from build123d import *

# Parameters (mm, degrees)
CROQUIS1_R              = 25.4
CROQUIS1_R_2            = 23.4
SALIENTE_EXTRUIR1_DEPTH = 1350
CROQUIS2_R              = 4
CROQUIS2_W              = 2520
CROQUIS2_H              = 10
CORTAR_EXTRUIR1_DEPTH   = 1351.477811739


with BuildPart() as part:
    # Croquis1 → Saliente-Extruir1 (new, symmetric)
    with BuildSketch(Plane(origin=(0, 0, 0), x_dir=(0, 0, -1), z_dir=(1, 0, 0))):
        Circle(CROQUIS1_R)
        Circle(CROQUIS1_R_2, mode=Mode.SUBTRACT)
    extrude(amount=SALIENTE_EXTRUIR1_DEPTH, both=True)

    # Croquis2 → Cortar-Extruir1 (cut, through all)
    with BuildSketch(Plane.XY):
        with Locations((-1339.465777124, 0)):
            Circle(CROQUIS2_R)
        Rectangle(CROQUIS2_W, CROQUIS2_H)
    extrude(amount=-CORTAR_EXTRUIR1_DEPTH, mode=Mode.SUBTRACT)


solid = part.part
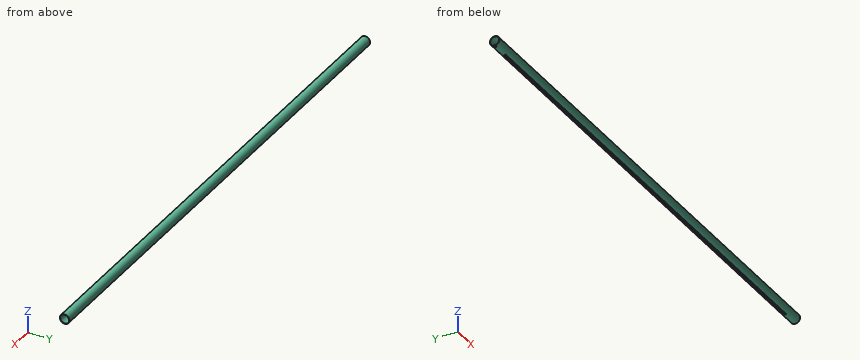
Geometry check sheet. Reference: the model listing, model coordinates, mm. Give positions to 0.01 mm unless a question says otherwise; leave off trailing zeros. Loops run counter-clockwise (first coordinate to the right, second up) from the corner with the lowest first, then second, coordinate; pieces in that order, holes last. Notation, with made-up numbers: M 84.25,65 L 106.25,65 A22 cw 106.25,99 Z; hole C 85.25,-36 d9. An arc over 180 degrees is marked long. Write each question's results on one line, items separated by ' | '.
1) Thickness scan on line 1 (X direction, y = 0, z = -24); line 2 (Y direction, x = -329, z = 0); line 3 (Z direction, x = 577.5, y = 13.5). Record the ranges inside material, lowest first.
Answers follow:
line 1: -1350 to -1343.47, -1335.47 to -1260, 1260 to 1350 | line 2: -25.4 to -23.4, 23.4 to 25.4 | line 3: -21.52 to -19.11, 19.11 to 21.52
2) Section check C-C, the plane x = -113. Record the boundary of the cut face in (y, z).
Answers follow:
outline: M -5,-24.9 L -5,-22.86 A23.4 cw long 5,-22.86 L 5,-24.9 A25.4 ccw long Z
3) Section check A-A, the plane z = 0. Record the boundary of the cut face in (x, y).
Answers follow:
outline: M -1350,-25.4 L 1350,-25.4 L 1350,-23.4 L -1350,-23.4 Z; M -1350,23.4 L 1350,23.4 L 1350,25.4 L -1350,25.4 Z
4) Gauge pin test, flat ends, axial feed: pin 1 (2 mm diameter, centred on x = -78.5, z = -24, fed in from -Y); pin 2 (3 mm diameter, centred on x = -148.5, z = 17.5, fed in from +Y); pin 3 (5 mm diameter, centred on x = 606.5, y = 4.5, fed in from -Z). Record the tip position at first contact, or that the pin passes through.
Answers follow:
pin 1: y = -10.78 | pin 2: y = 19.73 | pin 3: z = -24.9
5) Section check B-B, the plane y = 15.5. Record the boundary of the cut face in (x, z).
Answers follow:
outline: M -1350,-20.12 L 1350,-20.12 L 1350,-17.53 L -1350,-17.53 Z; M -1350,17.53 L 1350,17.53 L 1350,20.12 L -1350,20.12 Z
